Autodesk Inventor part; units mm, degrees
ref_plane "Start Plane" through (0, 0, 0) normal (1, 0, 0) x (0, 1, 0)
ref_plane "XZ Plane" through (0, 0, 0) normal (0, 1, 0) x (-1, 0, 0)
ref_plane "XY Plane" through (0, 0, 0) normal (0, 0, 1) x (1, 0, 0)
sketch "Main Sketch" plane through (0, 0, 0) normal (0, 0, 1) x (1, 0, 0)
  line L0 (0, 0) -> (238, 0)
  line L1 (0, 0) -> (0, 18)
  line L2 (0, 18) -> (58, 18)
  line L3 (58, 18) -> (58, 34)
  line L4 (76, 34) -> (76, 40)
  line L5 (58, 34) -> (76, 34)
  line L6 (136, 40) -> (136, 20)
  line L7 (76, 40) -> (136, 40)
  line L8 (156, 20) -> (156, 15)
  line L9 (136, 20) -> (156, 20)
  line L10 (181, 15) -> (181, 12.5)
  line L11 (156, 15) -> (181, 15)
  line L12 (238, 12.5) -> (238, 0)
  line L13 (181, 12.5) -> (238, 12.5)
  dimension "d3" = 36
  dimension "d4" = 68
  dimension "d5" = 80
  dimension "d6" = 40
  dimension "d7" = 30
  dimension "d8" = 25
revolve "Revolution1" add sketch "Main Sketch" angle 360 about axis through (0, 0, 0) along (1, 0, 0)
chamfer "Chamfer1" distance 2 angle 45 1 edges at (0, -18, 0) measured on face at (38.6667, 17.7669, -2.8874)
chamfer "Chamfer2" distance 2 angle 45 1 edges at (238, -12.5, 0) measured on face at (219, 12.4595, -1.0058)
equation "\"Length\" = 238"
properties part number "Shaft" material "Steel"
Verification items for the finished model (mm, model axes). A direction names the side the tool comes from. Round coordinates to 2 decimals unless told otherwise and drop trailing zeros. Order: outer loops, then holes, each group sorted by start corner. A loop starts at its lowest first (then second) coordinate and runs counter-clockwise, first axis right, second up.
1) Tool access check on faces 1 (the flat face through (58, 15, -15)), 2 (the cylindrical face through (208.885, 11.923, 3.755)), 3 (the cylindrical face through (106.42, -8.67, -39.05)). Record the directions out of +Z, -Z, +X, -X, +Y, -Y that give a thin tool (end or side, any length) a straight path to the whole face; none if there is none.
Geometry says:
face 1: -X
face 2: +X
face 3: +X, -X
2) Depth check by flat-ended pin: pin 1 (3 mm diameter, centred on x = 134, y = 21, fed in from +Z); pin 2 (12 mm diameter, centred on x = 44.5, z = 3, fed in from +Y); pin 3 (4 mm diameter, centred on y = -3.5, z = -24, fed in from -X). Enter the tip coordinate at first touch or a pass-through.
Geometry says:
pin 1: stops at z = 34.92
pin 2: stops at y = 18
pin 3: stops at x = 58
3) Cross-section at C-C, the plane x = 188. Record the cut outline in (y, z).
Geometry says:
outline: circle Ø25 at (0, 0)
4) Material ranges on line 1 (X direction, y = 22, z = 11); line 2 (X direction, y = 36.5, z = -14); line 3 (Y direction, x = 142, z = -12), recorded low to high.
Geometry says:
line 1: x = 58 to 136
line 2: x = 76 to 136
line 3: y = -16 to 16
5) Cross-section at A-A, the plane z = 0. Record the cut outline in (x, y).
Geometry says:
outline: (0, -16) - (2, -18) - (58, -18) - (58, -34) - (76, -34) - (76, -40) - (136, -40) - (136, -20) - (156, -20) - (156, -15) - (181, -15) - (181, -12.5) - (236, -12.5) - (238, -10.5) - (238, 10.5) - (236, 12.5) - (181, 12.5) - (181, 15) - (156, 15) - (156, 20) - (136, 20) - (136, 40) - (76, 40) - (76, 34) - (58, 34) - (58, 18) - (2, 18) - (0, 16) - close
6) Cross-section at D-D, the plane z = -26. Record the cut outline in (x, y), plus the area to 3 significant figures.
Geometry says:
outline: (58, -21.91) - (76, -21.91) - (76, -30.4) - (136, -30.4) - (136, 30.4) - (76, 30.4) - (76, 21.91) - (58, 21.91) - close
area: 4,440 mm2
